Could you check a few things on this model? Use its own coordinates, in mm. Face numbers are marked on the shaded views. Round coordinates to 2 decimals unless told otherwise and drop trailing zeros. Loops run counter-clockwise (first coordinate to the right, second up) from the corner with the lowest first, then second, coordinate; pieces in that order, holes last. Notation, with made-up numbers: (48.5, -4) -> (105.5, -4) arc R15 cw to (105.5, 10) -> close; hole circle Ø2 at (80.5, 39). An arc over 180 degrees is marked (long way). One line per item, written item: value.
```python
from build123d import *

# Parameters (mm, degrees)
SKETCH1_R           = 15.24
BOSS_EXTRUDE1_DEPTH = 68.58
SKETCH2_R           = 14.605
CUT_EXTRUDE1_DEPTH  = 68.58
SKETCH3_R           = 12.065
CUT_EXTRUDE2_DEPTH  = 68.58


with BuildPart() as part:
    # Sketch1 → Boss-Extrude1 (new body)
    with BuildSketch(Plane(origin=(0, 0, 0), x_dir=(1, 0, 0), z_dir=(0, 1, 0))):
        Circle(SKETCH1_R)
    extrude(amount=BOSS_EXTRUDE1_DEPTH)

    # Sketch2 → Cut-Extrude1 (cut)
    with BuildSketch(Plane.XY):
        with Locations((0, 35.56)):
            Circle(SKETCH2_R)
    extrude(amount=-CUT_EXTRUDE1_DEPTH, mode=Mode.SUBTRACT)

    # Sketch3 → Cut-Extrude2 (cut)
    with BuildSketch(Plane(origin=(0, 68.58, 0), x_dir=(-1, 0, 0), z_dir=(0, 1, 0))):
        Circle(SKETCH3_R)
    extrude(amount=-CUT_EXTRUDE2_DEPTH, mode=Mode.SUBTRACT)


solid = part.part
```
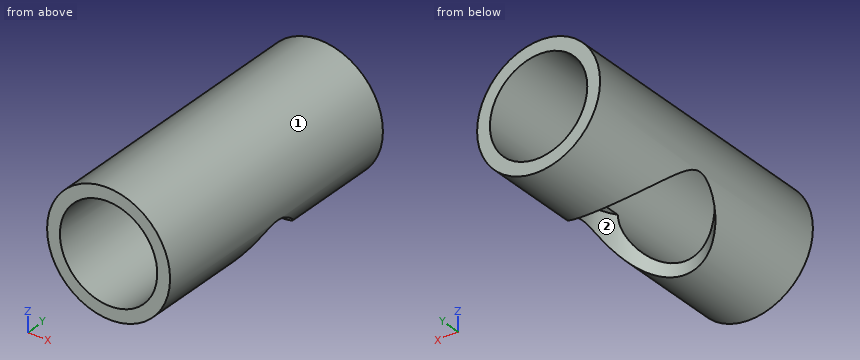
Item 1: I need wall thicknesses on line 1 (X direction, y = 50, z = 0) (3 decimals); line 2 (X direction, y = 23, z = -2). Which ranges of each line are inside material? Lowest first, please. Write a range as from..to.
Output:
line 1: x = -15.24..-12.065, 12.065..15.24
line 2: x = -15.11..-11.9, 11.9..15.11
Item 2: If we section it at C-C on y = 35.56: List the corners of the cut face in (x, z) for me (3 decimals), plus the area to 3 significant figures.
Output:
outline: (-14.605, -4.353) -> (-14.605, 0) -> (-12.065, 0) arc R12.065 cw to (12.065, 0) -> (14.605, 0) -> (14.605, -4.353) arc R15.24 ccw (long way) to start
area: 140 mm²
Item 3: If we mould it in two halves opening along X, with no side actions, what happens to the marked faces 1 and 2? For each: released by +X, released by -X, zero draft, split by the parting line, or undercut.
Output:
face 1: split by the parting line
face 2: undercut
Item 4: If we section it at A-A on x = 0: List the corners of the cut face in (y, z) for me (3 decimals), plus the area to 3 significant figures.
Output:
outline: (0, -15.24) -> (20.955, -15.24) -> (20.955, -12.065) -> (0, -12.065) -> close; (0, 12.065) -> (68.58, 12.065) -> (68.58, 15.24) -> (0, 15.24) -> close; (50.165, -15.24) -> (68.58, -15.24) -> (68.58, -12.065) -> (50.165, -12.065) -> close
area: 343 mm²
Item 5: If we section it at D-D on y = 23.5: List the corners of the cut face in (x, z) for me (3 decimals).
Output:
outline: (-8.238, -12.822) -> (-8.238, -8.815) arc R12.065 cw (long way) to (8.238, -8.815) -> (8.238, -12.822) arc R15.24 ccw (long way) to start
Item 6: If we section it at B-B on y = 7: List the corners of the cut face in (x, z) for me (3 decimals).
Output:
outline: circle Ø30.48 at (0, 0); hole circle Ø24.13 at (0, 0)
Item 7: Will these pins go through, and if not, where does the flat tip stop? pin 1 Ø8 at (x, y) = (9, 39) entering from +Z; pin 2 Ø1 at (y, z) = (29.5, 9) entering from +X; pin 3 Ø5 at (y, z) = (16, -3) entering from +X; pin 4 Ø4 at (x, z) = (1.5, 9) entering from +Y (3 decimals).
Output:
pin 1: stops at z = 14.4
pin 2: stops at x = 12.65
pin 3: stops at x = 15.23
pin 4: passes through
